Check sheet for the modelled part. Datum: model origin and axes. Units: mm. A direction names the side the tool comes from. Round coordinates to 2 decimals unless told otherwise and drop trailing zeros. Order: outer loops, then holes, each group sorted by start corner. A loop starts at its lowest first (then second) coordinate and runs counter-clockwise, first axis right, second up.
Q1. Cross-section at D-D on y = 0. Record the cut outline in (x, z), then the cut area to 3 significant figures.
Q2. Cross-section at C-C on x = -51. Record the cut outline in (y, z).
Q3. Scan lines: probe 1 along Z at (x, y) = (-9, -79); probe 2 along Z at (x, y) = (-15, -79); probe 3 along Z at (x, y) = (3, 70). Record each from-to range of solid material in increasing order.
Q4. Set-up check for faces 1 (the flat face through (0, -61, 15)), 2 (the flat face through (-10, 74, 15)), 3 (the flat face through (-12, -82, 10)), 4 (the flat face through (-5, 64.23, 4)): record each of +Z, -Z, +X, -X, +Y, -Y from which the full face is reachable in a straight line by a thin tool's end or side.
Q5. Cross-section at B-B on z = 15. Record the cut outline in (x, y), then the cut area to 3 significant figures.
Q6. Depth check by flat-ended pin: P1, Ø15, axis at y = -82, z = 21, coming from the +X side; P2, Ø3, axis at y = 8, z = 22.5, coming from the -X side; P3, Ø1, axis at y = -50.5, z = 5.5, coming from the +X side. Enter the tip coordinate at first touch or a pass-through.
Q7. Cross-section at A-A on y = -79.23. Record the cut outline in (x, z).
Q8. Mould release check, pull along Y, two halves, no side actions. Record for faces 5 (the cylindrical face through (-57.486, -1.264, 14.79)), 6 (the cylindrical face through (-64.958, 2.341, 14.79)), 7 (the flat face through (-17, -68, 11)), 8 (the flat face through (-5, 64.23, 26)): +Y half, -Y half, draft (parallel to the pull), parting line (faces both ways), or undercut.
from build123d import *

# Parameters (mm, degrees)
SKETCH_R        = 4
PAD_DEPTH       = 30
SKETCH001_R     = 5.5
POCKET_DEPTH    = 10
SKETCH002_R     = 11.5
POCKET001_DEPTH = 5
SKETCH003_R     = 1.75
POCKET002_DEPTH = 22.001
SKETCH005_W     = 20
SKETCH005_H     = 7.5
POCKET004_DEPTH = 20.001


with BuildPart() as body:
    # Sketch → Pad (new body)
    with BuildSketch(Plane.XY):
        with BuildLine():
            ThreePointArc((0, -57.5), (57.5, 0), (0, 57.5))
            Line((0, 64.226163), (0, 57.5))
            ThreePointArc((0, 84.226163), (-10, 74.226163), (0, 64.226163))
            Line((0, 84.226163), (10, 84.226163))
            Line((10, 84.226163), (10, 64.226163))
            ThreePointArc((17, -62.737549), (64.901433, 3.578267), (10, 64.226163))
            Line((17, -62.737549), (17, -94.226163))
            Line((17, -94.226163), (7, -94.226163))
            Line((7, -94.226163), (7, -64.226163))
            Line((7, -64.226163), (0, -64.226163))
            Line((0, -57.5), (0, -64.226163))
        make_face()
        with Locations((0, 74.226163)):
            Circle(SKETCH_R, mode=Mode.SUBTRACT)
    extrude(amount=PAD_DEPTH)

    # Sketch001 (on Face9 of Pad) → Pocket (cut)
    with BuildSketch(Plane(origin=(7, 0, 0), x_dir=(0, -1, 0), z_dir=(-1, 0, 0))):
        with Locations((79.23, 15)):
            Circle(SKETCH001_R)
    extrude(amount=-POCKET_DEPTH, mode=Mode.SUBTRACT)

    # Sketch002 (on Face11 of Pocket) → Pocket001 (cut)
    with BuildSketch(Plane.YZ.offset(17)):
        with Locations((-79.23, 15)):
            Circle(SKETCH002_R)
    extrude(amount=-POCKET001_DEPTH, mode=Mode.SUBTRACT)

    # Sketch003 (on Face17 of Pocket001) → Pocket002 (cut, through all)
    with BuildSketch(Plane.YZ.offset(12)):
        with Locations((-87.23, 15)):
            Circle(SKETCH003_R)
        with Locations((-79.23, 23)):
            Circle(SKETCH003_R)
        with Locations((-71.23, 15)):
            Circle(SKETCH003_R)
        with Locations((-79.23, 7)):
            Circle(SKETCH003_R)
    extrude(amount=-POCKET002_DEPTH, mode=Mode.SUBTRACT)

    # Sketch005 (on Face9 of Pocket002) → Pocket004 (cut, through all)
    with BuildSketch(Plane.YZ.offset(10)):
        with Locations((74.23, 26.25)):
            Rectangle(SKETCH005_W, SKETCH005_H)
        with Locations((74.23, 3.75)):
            Rectangle(SKETCH005_W, SKETCH005_H)
    extrude(amount=-POCKET004_DEPTH, mode=Mode.SUBTRACT)


with BuildPart() as part_mirroring:
    # Part__Mirroring: instance of Body
    add(body.part.mirror(Plane(origin=(0, 0, 0), x_dir=(0, -1, 0), z_dir=(1, 0, 0))))


solid = part_mirroring.part
Results found:
1. outline: (-65, 0) - (-57.5, 0) - (-57.5, 30) - (-65, 30) - close
1. area: 225 mm2
2. outline: (-40.3, 0) - (-26.56, 0) - (-26.56, 30) - (-40.3, 30) - close; (26.56, 0) - (40.3, 0) - (40.3, 30) - (26.56, 30) - close
3. probe 1: z = 0 to 5.27, 8.73 to 9.5, 20.5 to 21.27, 24.73 to 30
3. probe 2: z = 0 to 3.5, 26.5 to 30
3. probe 3: z = 7.5 to 22.5
4. face 1: +Z, -Z, +X, -Y
4. face 2: +Z, -Z, -X, +Y
4. face 3: -X
4. face 4: -Z, +X, -X, +Y
5. outline: (-17, -94.23) - (-7, -94.23) - (-7, -88.98) - (-12, -88.98) - (-12, -90.73) - (-17, -90.73) - close; (-17, -67.73) - (-12, -67.73) - (-12, -69.48) - (-7, -69.48) - (-7, -64.23) - (0, -64.23) - (0, -57.5) arc R57.5 cw to (0, 57.5) - (0, 64.23) arc R10 ccw to (0, 84.23) - (-10, 84.23) - (-10, 64.23) arc R65 ccw to (-17, -62.74) - close; (-12, -85.48) - (-7, -85.48) - (-7, -84.73) - (-12, -84.73) - close; (-12, -73.73) - (-7, -73.73) - (-7, -72.98) - (-12, -72.98) - close; hole circle Ø8 at (0, 74.23)
5. area: 1,840 mm2
6. P1: stops at x = -7
6. P2: stops at x = -64.67
6. P3: stops at x = -26.56
7. outline: (-17, 0) - (-7, 0) - (-7, 5.25) - (-12, 5.25) - (-12, 3.5) - (-17, 3.5) - close; (-17, 26.5) - (-12, 26.5) - (-12, 24.75) - (-7, 24.75) - (-7, 30) - (-17, 30) - close; (-12, 8.75) - (-7, 8.75) - (-7, 9.5) - (-12, 9.5) - close; (-12, 20.5) - (-7, 20.5) - (-7, 21.25) - (-12, 21.25) - close
8. face 5: undercut
8. face 6: parting line
8. face 7: draft
8. face 8: +Y half
